Read the model definition and answer for the solid it produces. Units are mm, in the model's axes. A direction names the side the tool comes from. Coordinates: 2 decimals unless noted, no trailing zeros. Loops run counter-clockwise (first coordinate to the right, second up) from the corner with the lowest first, then second, coordinate; pieces in that order, holes last. Notation, with made-up numbers: (84.5, 40.25) -> (131.5, 40.25) arc R31 ccw to (131.5, 70.25) -> close; hole circle Ø9 at (7.25, -3). An arc over 180 degrees is marked (long way). Answer as a JSON object with one key per item and string values. Group by question number.
Q1. The part is cut by section D-D on y = -158. Write down the section's boundary in (x, z), and give its area (3 significant figures).
Q2. The part is cut by section A-A on x = 4.1. Write down the section's boundary in (y, z), and give its area (3 significant figures).
Q3. Straight lines are drawn through the part: line 1 along Z through (x, y) = (2.2, -110); line 2 along Z through (x, y) = (2.3, -85); line 3 along Z through (x, y) = (1.1, -110). For each, find the intervals that lie inside material, in ascending order. Write a range as [from, to].
Q4. The part is cut by section B-B on y = -110. Write down the section's boundary in (x, z).
Q5. The part is cut by section C-C on y = -45. Write down the section's boundary in (x, z), and give its area (3 significant figures).
Q6. Each of these flat-tipped pins is pushed along its axis until it touches: P1, Ø2.5, axis at x = 1.5, y = -62.5, coming from the +Z side; P2, Ø4.5, axis at y = -35, z = 4, coming from the -X side; P3, Ø1.5, axis at x = 2.5, z = 7.5, coming from the -Y side; P4, Ø2, axis at y = -93.5, z = 12.5, coming from the -X side. Where does it stop, or does it pass through?
Q7. Determine the mould class of faces 1 (the flat face through (5.75, -158, 13)), 2 (the cylindrical face through (1.479, -137.718, 4.856)), 3 (the flat face through (3, -167, 4)) for opening direction Z: released by +Z, released by -Z, zero draft, split by the parting line, or undercut.
Q8. For faces 4 (the flat face through (2.3, -160, 7.6)), 5 (the flat face through (3, -62, 4)), 6 (the cylindrical face through (3, -158, 15)), determine the directions among +Z, -Z, +X, -X, +Y, -Y from which every point of the face is accessible in a straight line to the end or side of a thin tool.
from build123d import *

# Parameters (mm, degrees)
F1_DEPTH  = 5.75
F2_W      = 160
F2_H      = 0.9
F3_DEPTH  = 4.1
F5_DEPTH  = 3.5
F6_R      = 1.7
F7_DEPTH  = 25
F8_R      = 2.85
F8_R_2    = 1.7
F9_DEPTH  = 3
F11_DEPTH = 3.5
F12_W     = 2
F12_H     = 160
F12_W_2   = 3.75
F13_DEPTH = 2
F15_DEPTH = 5.75
F17_DEPTH = 25


# Not quite as in the source:
# - a feature names something its author has since deleted; it is built from what else it names


with BuildPart() as f1:
    # F0 (on Right) → F1 (new body)
    with BuildSketch(Plane.YZ):
        Polygon((-156, 10), (-160, 10), (-160, 0), (0, 0), (0, 10), align=None)
        with BuildLine():
            Line((-160, 13), (-160, 10))
            Line((-160, 10), (-156, 10))
            Line((-156, 10), (-156, 13))
            ThreePointArc((-156, 13), (-156.5857864376, 14.4142135624), (-158, 15))
            ThreePointArc((-158, 15), (-159.4142135624, 14.4142135624), (-160, 13))
        make_face()
    extrude(amount=F1_DEPTH)

    # F2 (on face) → F3 (cut)
    with BuildSketch(Plane.YZ.offset(5.75)):
        with Locations((-80, 8.55)):
            Rectangle(F2_W, F2_H)
    extrude(amount=-F3_DEPTH, mode=Mode.SUBTRACT)

    # F4 (on face) → F5 (cut)
    with BuildSketch(Plane.YZ.offset(5.75)):
        with BuildLine():
            ThreePointArc((-156, 13), (-158, 15), (-160, 13))
            Line((-160, 13), (-160, 9))
            Line((-160, 9), (0, 9))
            Line((0, 9), (0, 10))
            Line((0, 10), (-156, 10))
            Line((-156, 10), (-156, 13))
        make_face()
    extrude(amount=-F5_DEPTH, mode=Mode.SUBTRACT)

    # F6 (on face) → F7 (cut)
    with BuildSketch(Plane(origin=(0, 0, 0), x_dir=(0, -1, 0), z_dir=(-1, 0, 0))):
        with Locations((135, 4)):
            Circle(F6_R)
        with Locations((110, 4)):
            Circle(F6_R)
        with Locations((85, 4)):
            Circle(F6_R)
        with Locations((60, 4)):
            Circle(F6_R)
        with Locations((35, 4)):
            Circle(F6_R)
        with Locations((10, 4)):
            Circle(F6_R)
    extrude(amount=-F7_DEPTH, mode=Mode.SUBTRACT)

    # F8 (on face) → F9 (cut)
    with BuildSketch(Plane(origin=(0, 0, 0), x_dir=(0, -1, 0), z_dir=(-1, 0, 0))):
        with Locations((135, 4)):
            Circle(F8_R)
        with Locations((135, 4)):
            Circle(F8_R_2, mode=Mode.SUBTRACT)
        with Locations((110, 4)):
            Circle(F8_R)
        with Locations((110, 4)):
            Circle(F8_R_2, mode=Mode.SUBTRACT)
        with Locations((85, 4)):
            Circle(F8_R)
        with Locations((85, 4)):
            Circle(F8_R_2, mode=Mode.SUBTRACT)
        with Locations((60, 4)):
            Circle(F8_R)
        with Locations((60, 4)):
            Circle(F8_R_2, mode=Mode.SUBTRACT)
        with Locations((35, 4)):
            Circle(F8_R)
        with Locations((35, 4)):
            Circle(F8_R_2, mode=Mode.SUBTRACT)
        with Locations((10, 4)):
            Circle(F8_R)
        with Locations((10, 4)):
            Circle(F8_R_2, mode=Mode.SUBTRACT)
    extrude(amount=-F9_DEPTH, mode=Mode.SUBTRACT)

    # F10 (on face) → F11 (join, through all)
    with BuildSketch(Plane.YZ.offset(2.25)):
        with BuildLine():
            ThreePointArc((-160, 13), (-158, 11), (-156, 13))
            ThreePointArc((-156, 13), (-158, 15), (-160, 13))
        make_face()
    extrude(amount=F11_DEPTH)

    # F12 (on face) → F13 (join)
    with BuildSketch(Plane(origin=(0, 0, 0), x_dir=(1, 0, 0), z_dir=(0, 0, -1))):
        with Locations((1, 80)):
            Rectangle(F12_W, F12_H)
        with Locations((3.875, 80)):
            Rectangle(F12_W_2, F12_H)
    extrude(amount=F13_DEPTH)

    # F14 (on face) → F15 (join, through all)
    with BuildSketch(Plane.YZ.offset(5.75)):
        Polygon((-175, 0), (-160, 0), (-160, 4), (-163, 4), (-163, 1.9), (-165.1, 1.9), (-165.1, 4), (-169, 4), (-169, 1.9), (-171.1, 1.9), (-171.1, 4), (-175, 4), align=None)
    extrude(amount=-F15_DEPTH)

    # F16 (on face) → F17 (cut)
    with BuildSketch(Plane.YZ.offset(5.75)):
        Polygon((-2, 0), (0, 0), (0, 3.1547005384), (-2, 2), align=None)
    extrude(amount=-F17_DEPTH, mode=Mode.SUBTRACT)


solid = f1.part
Final values:
{
 "1": {"outline": "(0, -2) -> (5.75, -2) -> (5.75, 8.1) -> (1.65, 8.1) -> (1.65, 9) -> (2.25, 9) -> (2.25, 11) -> (5.75, 11) -> (5.75, 15) -> (0, 15) -> close", "area": "87.1 mm2"},
 "2": {"outline": "(-175, 0) -> (-160, 0) -> (-160, -2) -> (0, -2) -> (0, 0) -> (-2, 0) -> (-2, 2) -> (0, 3.15) -> (0, 8.1) -> (-160, 8.1) -> (-160, 4) -> (-163, 4) -> (-163, 1.9) -> (-165.1, 1.9) -> (-165.1, 4) -> (-169, 4) -> (-169, 1.9) -> (-171.1, 1.9) -> (-171.1, 4) -> (-175, 4) -> close; circle Ø4 at (-158, 13); hole circle Ø3.4 at (-135, 4); hole circle Ø3.4 at (-110, 4); hole circle Ø3.4 at (-85, 4); hole circle Ø3.4 at (-60, 4); hole circle Ø3.4 at (-35, 4); hole circle Ø3.4 at (-10, 4)", "area": "1,620 mm2"},
 "3": {"line 1": "z = [-2, 1.15], [6.85, 8.1], [9, 10]", "line 2": "z = [-2, 1.15], [6.85, 8.1]", "line 3": "z = [-2, 1.15], [6.85, 10]"},
 "4": {"outline": "(0, -2) -> (5.75, -2) -> (5.75, 2.3) -> (3, 2.3) -> (3, 1.15) -> (0, 1.15) -> close; (0, 6.85) -> (3, 6.85) -> (3, 5.7) -> (5.75, 5.7) -> (5.75, 8.1) -> (1.65, 8.1) -> (1.65, 9) -> (2.25, 9) -> (2.25, 10) -> (0, 10) -> close"},
 "5": {"outline": "(0, -2) -> (5.75, -2) -> (5.75, 8.1) -> (1.65, 8.1) -> (1.65, 9) -> (2.25, 9) -> (2.25, 10) -> (0, 10) -> close", "area": "61.8 mm2"},
 "6": {"P1": "stops at z = 10", "P2": "stops at x = 3", "P3": "stops at y = -160", "P4": "passes through"},
 "7": {"face 1": "zero draft", "face 2": "undercut", "face 3": "released by +Z"},
 "8": {"face 4": "+Z, +X, -X, -Y", "face 5": "-X", "face 6": "+X"}
}
